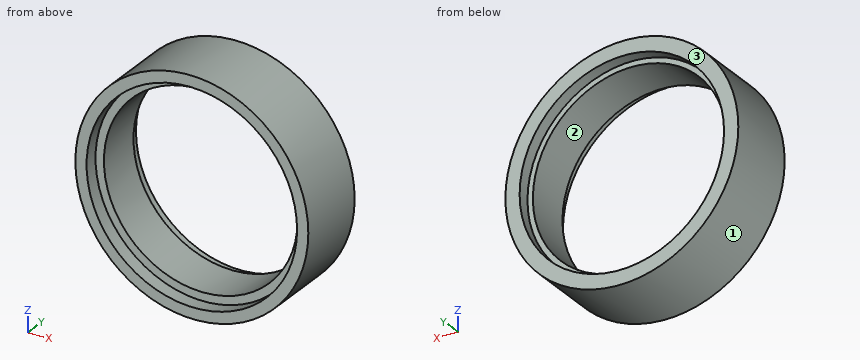
from build123d import *

# Parameters (mm, degrees)
F0_R     = 21.082
F0_R_2   = 17.526
F1_DEPTH = 13
F2_R     = 19.05
F3_DEPTH = 2.5
F4_R     = 18.5
F5_DEPTH = 2.2


with BuildPart() as f1:
    # F0 (on Front) → F1 (new body)
    with BuildSketch(Plane.XZ):
        Circle(F0_R)
        Circle(F0_R_2, mode=Mode.SUBTRACT)
    extrude(amount=F1_DEPTH)

    # F2 (on face) → F3 (cut)
    with BuildSketch(Plane.XZ.offset(13)):
        Circle(F2_R)
    extrude(amount=-F3_DEPTH, mode=Mode.SUBTRACT)

    # F4 (on face) → F5 (cut)
    with BuildSketch(Plane(origin=(0, 0, 0), x_dir=(-1, 0, 0), z_dir=(0, 1, 0))):
        Circle(F4_R)
    extrude(amount=-F5_DEPTH, mode=Mode.SUBTRACT)


solid = f1.part
Read the model definition and answer for the solid it produces. Units are mm, in the model's axes. Face numbers are marked on the shaded views. Coordinates: 2 decimals unless noted, no trailing zeros. Loops run counter-clockwise (first coordinate to the right, second up) from the corner with the lowest first, then second, coordinate; pieces in that order, holes last.
Q1. The mould has two halves that part along X. Classify the marked faces 1, 2 and 3: +X half, -X half, draft (parallel to the pull), parting line (faces both ways), or undercut.
Q2. The part is cut by section B-B on z = 0. Write down the section's boundary in (x, y), and give its area (3 significant figures).
Q3. Each of these flat-tipped pins is pushed along its axis until it touches: pin 1 Ø1 at (y, z) = (-2, -7.5) entering from -X; pin 2 Ø2 at (y, z) = (-4, -16) entering from -X; pin 3 Ø2 at (x, y) = (-4, -2) entering from +Z. Where does it stop, or does it pass through?
Q4. The part is cut by section A-A on x = 0. Write down the section's boundary in (y, z).
Q5. Consider probe 1 along Z at (x, y) = (0, -5.5); probe 2 along Z at (x, y) = (0, -0.45); probe 3 along X at (y, z) = (-6.5, 15.5). Determine where each line is inside the solid, lowest interval first.
Q6. The part is cut by section C-C on y = -6.25. Write down the section's boundary in (x, z), and give its area (3 significant figures).
Results below:
1. face 1: parting line
1. face 2: undercut
1. face 3: draft
2. outline: (-21.08, -13) - (-19.05, -13) - (-19.05, -10.5) - (-17.53, -10.5) - (-17.53, -2.2) - (-18.5, -2.2) - (-18.5, 0) - (-21.08, 0) - close; (17.53, -10.5) - (19.05, -10.5) - (19.05, -13) - (21.08, -13) - (21.08, 0) - (18.5, 0) - (18.5, -2.2) - (17.53, -2.2) - close
2. area: 80.6 mm2
3. pin 1: stops at x = -19.89
3. pin 2: stops at x = -14.81
3. pin 3: stops at z = 20.87
4. outline: (-13, -21.08) - (0, -21.08) - (0, -18.5) - (-2.2, -18.5) - (-2.2, -17.53) - (-10.5, -17.53) - (-10.5, -19.05) - (-13, -19.05) - close; (-13, 19.05) - (-10.5, 19.05) - (-10.5, 17.53) - (-2.2, 17.53) - (-2.2, 18.5) - (0, 18.5) - (0, 21.08) - (-13, 21.08) - close
5. probe 1: z = -21.08 to -17.53, 17.53 to 21.08
5. probe 2: z = -21.08 to -18.5, 18.5 to 21.08
5. probe 3: x = -14.29 to -8.18, 8.18 to 14.29
6. outline: circle Ø42.16 at (0, 0); hole circle Ø35.05 at (0, 0)
6. area: 431 mm2
